```python
from build123d import *

# Parameters (mm, degrees)
IZIM1_W                     = 58.4
IZIM1_H                     = 31.6
Y_KSEKLIK_EKSTR_ZYON1_DEPTH = 19
IZIM2_W                     = 58.4
IZIM2_H                     = 31.6
Y_KSEKLIK_EKSTR_ZYON2_DEPTH = 1.6
KES_EKSTR_ZYON2_START       = 59.6
KES_EKSTR_ZYON2_DEPTH       = 3


with BuildPart() as part:
    # Çizim1 → Yükseklik-Ekstrüzyon1 (new body)
    with BuildSketch(Plane.XY):
        Polygon((0, 32.8), (59.6, 32.8), (59.6, -1.2), (-1.6, -1.2), (-1.6, 32.8), align=None)
        with Locations((29.2, 15.8)):
            Rectangle(IZIM1_W, IZIM1_H, mode=Mode.SUBTRACT)
    extrude(amount=Y_KSEKLIK_EKSTR_ZYON1_DEPTH)

    # Çizim2 → Yükseklik-Ekstrüzyon2 (add)
    with BuildSketch(Plane.XY):
        with Locations((29.2, 15.8)):
            Rectangle(IZIM2_W, IZIM2_H)
    extrude(amount=Y_KSEKLIK_EKSTR_ZYON2_DEPTH)

    # Çizim3 → Kes-Ekstrüzyon2 (cut)
    with BuildSketch(Plane(origin=(0, 0, 0), x_dir=(0, 0, -1), z_dir=(1, 0, 0)).offset(KES_EKSTR_ZYON2_START)):
        Polygon((-1.790149403, 19.741982838), (-1.790149403, 11.741982838), (-5.27887078, 12.594196568), (-5.27887078, 18.754449839), align=None)
    extrude(amount=-KES_EKSTR_ZYON2_DEPTH, mode=Mode.SUBTRACT)


solid = part.part
```
For this review, take the finished solid that the model builds, in its own axes (mm). A direction names the side the tool comes from. Coordinates: 2 decimals unless noted, no trailing zeros. Loops run counter-clockwise (first coordinate to the right, second up) from the corner with the lowest first, then second, coordinate; pieces in that order, holes last. Notation, with made-up numbers: (50, 44.25) - (75, 44.25) arc R26 ccw to (75, 66.25) - close; hole circle Ø9 at (18.25, -38.75). An arc over 180 degrees is marked (long way). Use one line per item in the form item = value. Start each with the question number.
1) Take a section at D-D (y = 22). State the section outline as (x, z) points.
2) Take a section at A-A (y = 16.5). State the section outline as (x, z) points.
3) To check wall thickness, follow probe 1 along Y at (x, z) = (33, 13.75); probe 2 along X at (y, z) = (26, 8); probe 3 along Z at (x, y) = (24, 19). State the ranges of each line that lie inside material, in increasing order. Write a range as from..to.
4) Draft analysis for pull direction Y (two halves, no side actions). For faces 1 (the face through (29, 0, 10)), 2 (the face through (29, -1.2, 9)), 3 (the face through (29, 32.8, 9)), 4 (the face through (-1.6, 16, 9)), state which applies: released by +Y, released by -Y, zero draft, split by the parting line, or undercut.
5) For pin 1 (16 mm diameter, centred on x = 20.5, y = 9.5, fed in from +Z), flat-tipped, find the tip position at first contact; note if it passes through.
6) Take a section at B-B (z = 7.25). State the section outline as (x, y) points.
7) For faces 5 (the face through (58.4, 16, 10)), 6 (the face through (59, 16, 5.279)), 7 (the face through (29, 16, 0)), list the 3-axis set-ups (+Z, -Z, +X, -X, +Y, -Y) from which the entire face can be reached by the end or side of a thin tool; tool diameter is ignored.
8) Take a section at C-C (x = 52.5). State the section outline as (y, z) points, plus the area to 3 significant figures.
From the geometry:
q1.outline = (-1.6, 0) - (59.6, 0) - (59.6, 19) - (58.4, 19) - (58.4, 1.6) - (0, 1.6) - (0, 19) - (-1.6, 19) - close
q2.outline = (-1.6, 0) - (59.6, 0) - (59.6, 1.79) - (58.4, 1.79) - (58.4, 1.6) - (0, 1.6) - (0, 19) - (-1.6, 19) - close; (58.4, 5.28) - (59.6, 5.28) - (59.6, 19) - (58.4, 19) - close
q3.probe_1 = -1.2..0, 31.6..32.8
q3.probe_2 = -1.6..0, 58.4..59.6
q3.probe_3 = 0..1.6
q4.face_1 = undercut
q4.face_2 = released by -Y
q4.face_3 = released by +Y
q4.face_4 = zero draft
q5.pin_1 = 1.6
q6.outline = (-1.6, -1.2) - (59.6, -1.2) - (59.6, 32.8) - (-1.6, 32.8) - close; hole (0, 0) - (58.4, 0) - (58.4, 31.6) - (0, 31.6) - close
q7.face_5 = +Z
q7.face_6 = +X
q7.face_7 = -Z, +X, -X, +Y, -Y
q8.outline = (-1.2, 0) - (32.8, 0) - (32.8, 19) - (31.6, 19) - (31.6, 1.6) - (0, 1.6) - (0, 19) - (-1.2, 19) - close
q8.area = 96.2 mm2
